The drawing under review shows one solid part. Ordinate dimensions are in mm from its lowest x, y, z. A direction names the side the tool comes from. Coordinates: 2 decimals unless noted, no trailing zeros. Write each loop counter-clockwise with the first axis right and the second up, starting at its lowest first coordinate (ties: lowest second). Pieces come first, ordered by that corner, then holes. Notation, with made-up numbers: (64.5, 66.25) - (99.5, 66.25) arc R15 cw to (99.5, 91.25) - close; hole circle Ø11 at (-13, 70.5). An arc over 180 degrees is marked (long way). Put each result on its own line as item: value. Start each with the question number.
Item 1: Consider section D-D on z = 0.45. Give the boundary of the cut face in (x, y), then the cut area to 3 significant figures.
Item 2: Consider section A-A on y = 4. Give the boundary of the cut face in (x, z), then the cut area to 4 significant figures.
Item 3: To check wall thickness, follow L1, parallel to Y at x = 4, z = 2.6; L2, parallel to Y at x = 4, z = 0.8; L3, parallel to Z at x = 6.25, y = 5.5. State the ranges of each line that lie inside material, in increasing order. Write a range as [from, to].
Item 4: Machinability: for the marked faces 4 and 5, which of the approach directions +Z, -Z, +X, -X, +Y, -Y give a long, thin tool a straight path to every point of the face, cutting with its end or side? Answer none if there is none.
Item 5: For pin 1 (1.5 mm diameter, centred on y = 1, z = 2, fed in from -X), flat-tipped, find the tip position at first contact; note if it passes through.
Item 6: Consider section C-C on z = 1.15. Give the boundary of the cut face in (x, y).
Item 7: Mouldability with a two-part tool opening along X and no side actions: class the marked faces 1, 2 and 3 as pulls with the +X half, pulls with the -X half, needs draft (parallel to the pull), parting line crosses it, or undercut.
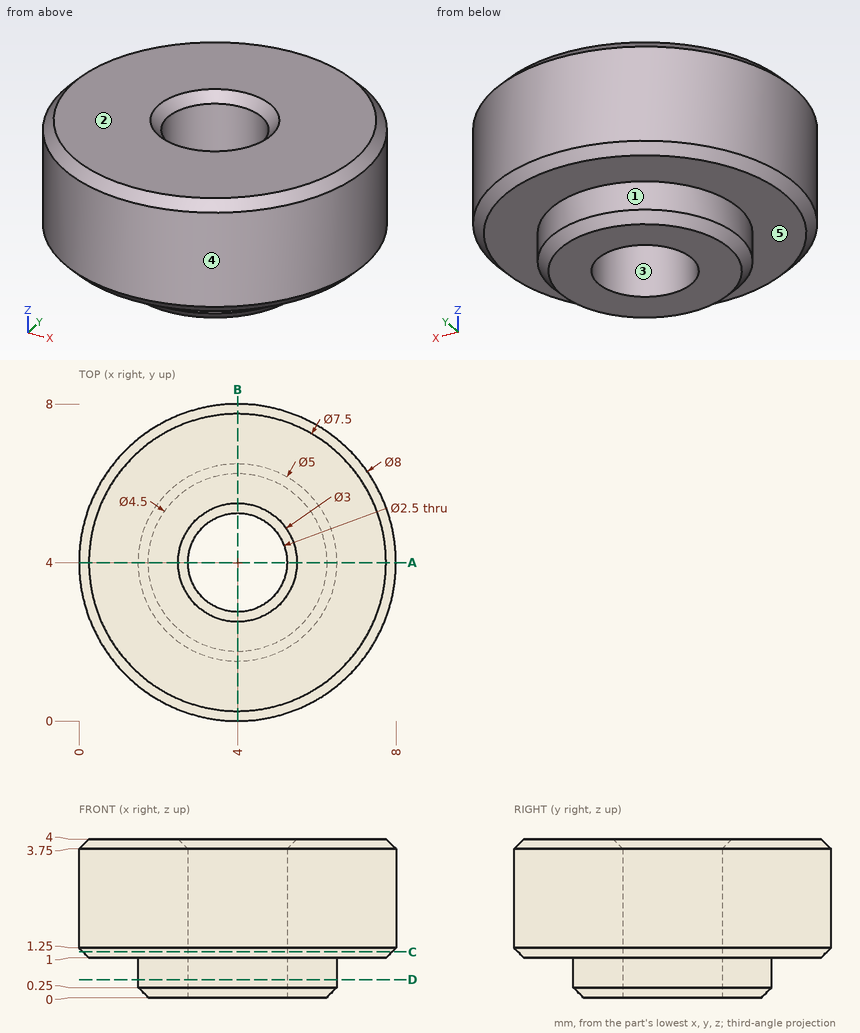
Report:
1. outline: circle Ø5 at (4, 4); hole circle Ø2.5 at (4, 4)
1. area: 14.7 mm²
2. outline: (0, 1.25) - (0.25, 1) - (1.5, 1) - (1.5, 0.25) - (1.75, 0) - (2.75, 0) - (2.75, 3.75) - (2.5, 4) - (0.25, 4) - (0, 3.75) - close; (5.25, 0) - (6.25, 0) - (6.5, 0.25) - (6.5, 1) - (7.75, 1) - (8, 1.25) - (8, 3.75) - (7.75, 4) - (5.5, 4) - (5.25, 3.75) - close
2. area: 18.75 mm²
3. L1: [0, 2.75], [5.25, 8]
3. L2: [1.5, 2.75], [5.25, 6.5]
3. L3: [1, 4]
4. face 4: +Z, -Z
4. face 5: -Z
5. pin 1: x = 0.69
6. outline: circle Ø7.8 at (4, 4); hole circle Ø2.5 at (4, 4)
7. face 1: parting line crosses it
7. face 2: needs draft
7. face 3: undercut
